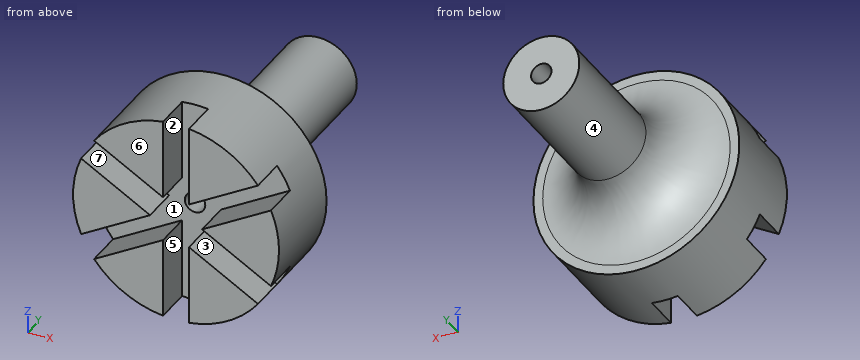
```python
from build123d import *

# Parameters (mm, degrees)
CORTE_EXTRUS_O2_DEPTH = 2
FILETE1_R             = 3


with BuildPart() as part:
    # Esboço1 → Revolução1 (revolve)
    with BuildSketch(Plane.XY):
        Polygon((0.55, 10), (2.05, 10), (2.05, 0), (5.55, 0), (5.55, -5), (0.55, -5), align=None)
    revolve(axis=Axis((0, 0, 0), (0, 1, 0)))

    # Esboço2 → Corte-extrusão2 (cut)
    with BuildSketch(Plane.XZ.offset(5)):
        Polygon((-0.7, 5.55), (-0.7, 1.212435565), (-4.456440991, 3.381217783), (-5.156440991, 2.168782217), (-1.4, 0), (-5.156440991, -2.168782217), (-4.456440991, -3.381217783), (-0.7, -1.212435565), (-0.7, -5.55), (0.7, -5.55), (0.7, -1.212435565), (4.456440991, -3.381217783), (5.156440991, -2.168782217), (1.4, 0), (5.156440991, 2.168782217), (4.456440991, 3.381217783), (0.7, 1.212435565), (0.7, 5.55), align=None)
    extrude(amount=-CORTE_EXTRUS_O2_DEPTH, mode=Mode.SUBTRACT)

    # Filete1
    filete1_edges = [part.edges().sort_by_distance(p)[0] for p in [
        (-2.05, 0, 0),
    ]]
    fillet(filete1_edges, radius=FILETE1_R)


solid = part.part
```
The listing builds one solid part. Answer for the finished solid, in the listing's coordinates (mm). Face numbers are marked on the shaded views. A direction names the side the tool comes from. Coordinates: 2 decimals unless noted, no trailing zeros. Write each loop counter-clockwise with the first axis right and the second up, starting at its lowest first coordinate (ties: lowest second). Pieces come first, ordered by that corner, then holes. Notation, with made-up numbers: M 18,67.5 L 36,67.5 A12 cw 36,76.5 Z; hole C 30,-31 d8. An arc over 180 degrees is marked long. Use a Markdown table: item, result. Add a question column.
1. Straight lines are drawn through the part: line 1 along Z through (x, y) = (0, 5.25); line 2 along Z through (x, y) = (-3, -3.5). For each, find the intervals that lie inside material, in ascending order. Write a range as [from, to].
2. Section A-A (x = 0) is taken. Give the vertices of the cut face in (y, z).
3. For a pull along Z with two mould halves and no side action, classify the marked faces 1, 2, 3 and 4 as +Z half, -Z half, draft (parallel to the pull), parting line (faces both ways), or undercut.
4. Section C-C (y = 1.5) is taken. Give the vertices of the cut face in (x, z).
5. Which of the six approach directions +Z, -Z, +X, -X, +Y, -Y give full straight-line access (tool end or side, diameter ignored) to the marked faces 5, 6 and 7?
6. Section B-B (y = 5.5) is taken. Give the vertices of the cut face in (x, z).
7. Given P1, Ø0.6, axis at y = -4, z = 3, coming from the -X side; P2, Ø1.5, axis at y = 8.5, z = -4, coming from the +X side; P3, Ø5, axis at x = 2.5, y = 3, coming from the +Z side; P4, Ø1.6, axis at y = -4, z = -3, coming from the +X side, each flat-ended and moving along its own axis, determine where each tip first touches the part or whether it passes through.
Data:
| question | item | result |
|---|---|---|
| 1 | line 1 | z = [-2.05, -0.55], [0.55, 2.05] |
| 1 | line 2 | z = [-4.67, -2.54], [-0.92, 0.92], [2.54, 4.67] |
| 2 | outline | M -3,-5.55 L 0,-5.55 L 0,-5.05 A3 cw 3,-2.05 L 10,-2.05 L 10,-0.55 L -3,-0.55 Z; M -3,0.55 L 10,0.55 L 10,2.05 L 3,2.05 A3 cw 0,5.05 L 0,5.55 L -3,5.55 Z |
| 3 | face 1 | undercut |
| 3 | face 2 | draft |
| 3 | face 3 | undercut |
| 3 | face 4 | parting line |
| 4 | outline | C 0,0 d4.9; hole C 0,0 d1.1 |
| 5 | face 5 | +Z, -Z, -Y |
| 5 | face 6 | +Z, -Z, +X, -X, -Y |
| 5 | face 7 | -Y |
| 6 | outline | C 0,0 d4.1; hole C 0,0 d1.1 |
| 7 | P1 | stops at x = -4.32 |
| 7 | P2 | passes through |
| 7 | P3 | stops at z = 2.73 |
| 7 | P4 | stops at x = 4.42 |
